Input: part model. Units: mm. Frame: model coordinates. A direction names the side the tool comes from. Coordinates: 2 decimals unless noted, no trailing zeros. Write each loop counter-clockwise with the first axis right and the second up, starting at its lowest first coordinate (ties: lowest second). Pieces come first, ordered by that corner, then holes. Notation, with made-up numbers: M 85,26.25 L 117,26.25 A25 ccw 117,49.25 Z; hole C 64.25,-26.75 d1. An arc over 180 degrees is marked long. Write each question's results on one line, items separated by ' | '. Start each with the question number.
1. Pull-direction query (Y, two-part tool) for faces 1 (the flat face through (-20, 40, 4)), 2 (the cylindrical face through (-19.97, 43.32, 5.48)), 3 (the flat face through (-19, 9, 15)), 4 (the flat face through (-20, 46.758, -2)); classes: +Y half, -Y half, draft (parallel to the pull), parting line (faces both ways), or undercut.
2. Set-up query: faces 5 (the flat face through (-19, 15, 7)), 6 (the flat face through (-6.358, 11.012, 1.972)), 7 (the flat face through (-22.814, 12, 6)), 8 (the flat face through (-20, 28.489, 5)). Return all of +Z, -Z, +X, -X, +Y, -Y with unobstructed straight access to the full face (end or side cutting, diameter ignored); none if empty.
3. Section query C-C, the plane y = 30. Output: boundary loops of the cut face in (x, z).
4. Section query B-B, the plane x = -11. Output: boundary loops of the cut face in (y, z), and give its area (3 significant figures).
5. Section query D-D, the plane x = -22. Output: boundary loops of the cut face in (y, z).
6. Section query A-A, the plane z = 1.25. Output: boundary loops of the cut face in (x, y), and give its area (3 significant figures).
7. Ray query, probe 1 along Z at (x, y) = (-29, 45.5); probe 2 along Y at (x, z) = (-6, -5.5); probe 3 along Z at (x, y) = (-27, 25.5). Return the intervals inside material, ascending.
8. First-contact query: pin 1 (22 mm diameter, centred on x = -12.5, y = 35.5, fed in from +Z); pin 2 (1.2 mm diameter, centred on x = -28.5, z = -1.5, fed in from -Y); pin 3 (12 mm diameter, centred on y = 16.5, z = 11.5, fed in from -X). Flat tips, straight axial feed; report the tip coordinate or a pass-through.
```python
from build123d import *

# Parameters (mm, degrees)
F1_DEPTH  = 4
F2_W      = 40
F2_H      = 3.4614801407
F3_DEPTH  = 8
F4_W      = 40
F4_H      = 4
F5_DEPTH  = 10
F6_W      = 7.1115158498
F6_H      = 16.9303966686
F7_DEPTH  = 3
F8_W      = 7.1115158498
F8_H      = 3.3362442628
F9_DEPTH  = 8
F10_W     = 7.1115158498
F10_H     = 4
F11_DEPTH = 5
F13_DEPTH = 3


with BuildPart() as f1:
    # F0 (on Top) → F1 (new body)
    with BuildSketch(Plane.XY):
        Polygon((-40, 0), (0, 0), (-12.8963018344, 22.337050007), (0, 34.6410161514), (0, 50.2190850675), (-40, 50.2190850675), (-40, 34.6410161514), (-27.1036981656, 22.337050007), align=None)
    extrude(amount=F1_DEPTH)

    # F2 (on face) → F3 (join)
    with BuildSketch(Plane(origin=(0, 0, 0), x_dir=(1, 0, 0), z_dir=(0, 0, -1))):
        with Locations((-20, -48.4883449972)):
            Rectangle(F2_W, F2_H)
    extrude(amount=F3_DEPTH)

    # F4 (on face) → F5 (join)
    with BuildSketch(Plane.XZ.offset(-46.7576049268)):
        with Locations((-20, -6)):
            Rectangle(F4_W, F4_H)
    extrude(amount=F5_DEPTH)

    # F6 (on face) → F7 (join)
    with BuildSketch(Plane.XY.offset(4)):
        with Locations((-19.2582923919, 13.6125446297)):
            Rectangle(F6_W, F6_H)
    extrude(amount=F7_DEPTH)

    # F8 (on face) → F9 (join)
    with BuildSketch(Plane.XY.offset(7)):
        with Locations((-19.2582923919, 6.8154684268)):
            Rectangle(F8_W, F8_H)
    extrude(amount=F9_DEPTH)

    # F10 (on face) → F11 (join)
    with BuildSketch(Plane(origin=(0, 8.4835905582, 0), x_dir=(-1, 0, 0), z_dir=(0, 1, 0))):
        with Locations((19.2582923919, 13)):
            Rectangle(F10_W, F10_H)
    extrude(amount=F11_DEPTH)

    # F12 (on face) → F13 (join)
    with BuildSketch(Plane.XY.offset(4)):
        Polygon((-20, 50.2190850675), (-26.4434188207, 39.887223703), (-26.5116588016, 39.7778025957), (-26.7759245414, 39.3540590733), (-33.5518490828, 28.4890330792), (-6.4481509172, 28.4890330792), (-13.2240754586, 39.3540590733), (-13.4883411984, 39.7778025957), align=None)
        with BuildLine():
            ThreePointArc((-26.3472255319, 40.0048010051), (-19.8613519763, 43.32080982), (-13.4933032095, 39.7838018835))
            ThreePointArc((-13.4933032095, 39.7838018835), (-19.9874553417, 35.9862880757), (-26.3472255319, 40.0048010051))
        make_face(mode=Mode.SUBTRACT)
    extrude(amount=F13_DEPTH)


solid = f1.part
```
Answer:
1) face 1: undercut | face 2: undercut | face 3: draft | face 4: -Y half
2) face 5: +X, -X, +Y | face 6: +Z, -Z, +X | face 7: +Z, -X, -Y | face 8: +Z, +X, -X
3) outline: M -35.14,0 L -4.86,0 L -4.86,4 L -7.39,4 L -7.39,7 L -32.61,7 L -32.61,4 L -35.14,4 Z
4) outline: M 0,0 L 19.05,0 L 19.05,4 L 0,4 Z; M 24.15,0 L 46.76,0 L 46.76,-4 L 36.76,-4 L 36.76,-8 L 50.22,-8 L 50.22,4 L 35.79,4 L 35.79,7 L 28.49,7 L 28.49,4 L 24.15,4 Z | area: 270 mm^2
5) outline: M 0,0 L 46.76,0 L 46.76,-4 L 36.76,-4 L 36.76,-8 L 50.22,-8 L 50.22,4 L 47.01,4 L 47.01,7 L 43.06,7 L 43.06,4 L 36.31,4 L 36.31,7 L 28.49,7 L 28.49,4 L 22.08,4 L 22.08,7 L 8.48,7 L 8.48,11 L 13.48,11 L 13.48,15 L 5.15,15 L 5.15,4 L 0,4 Z
6) outline: M -40,0 L 0,0 L -12.9,22.34 L 0,34.64 L 0,50.22 L -40,50.22 L -40,34.64 L -27.1,22.34 Z | area: 1,560 mm^2
7) probe 1: -8 to -4, 0 to 4 | probe 2: 36.76 to 50.22 | probe 3: 0 to 4
8) pin 1: z = 7 | pin 2: y = 46.76 | pin 3: x = -22.81
